Geometry check sheet. Reference: the model listing, model coordinates, mm. Face numbers are marked on the shaded views. A direction names the side the tool comes from. Coordinates: 2 decimals unless noted, no trailing zeros. Loops run counter-clockwise (first coordinate to the right, second up) from the corner with the lowest first, then second, coordinate; pieces in that order, holes last. Notation, with made-up numbers: M 12.5,-27 L 31.5,-27 A5 cw 31.5,-22 Z; hole C 66,-2 d8. An arc over 180 degrees is marked long. Use CSV: the item, a comma, the result in double quotes.
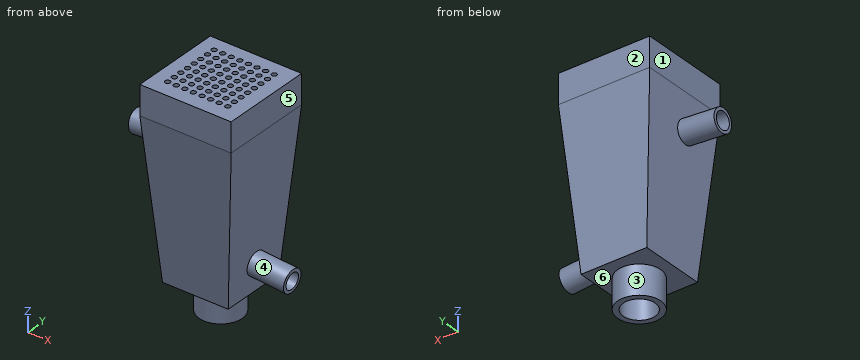
```python
from build123d import *

# Parameters (mm, degrees)
SKETCH2_4_W         = 25
SKETCH2_4_H         = 25
BOSS_EXTRUDE2_DEPTH = 8
SKETCH5_R           = 0.7
CUT_EXTRUDE1_DEPTH  = 8
SKETCH6_R           = 3.1
SKETCH6_R_2         = 2.3
BOSS_EXTRUDE4_DEPTH = 10
CUT_EXTRUDE2_START  = -4
SKETCH6_4_R         = 2.3
CUT_EXTRUDE2_DEPTH  = 4
SKETCH9_R           = 3.1
SKETCH9_R_2         = 2.2
BOSS_EXTRUDE5_DEPTH = 10
SKETCH1_7_R         = 5.88
SKETCH1_7_R_2       = 4.38
BOSS_EXTRUDE7_DEPTH = 8
CUT_EXTRUDE3_START  = -20
SKETCH10_R          = 2.2
CUT_EXTRUDE3_DEPTH  = 20


with BuildPart() as part:
    # Sketch1 → Loft1 section 0
    with BuildSketch(Plane.XY):
        with BuildLine():
            Line((-9, 9), (9, 9))
            Line((9, 9), (9, -9))
            Line((9, -9), (-9, -9))
            Line((-9, -9), (-9, 9))
        make_face()
    # Sketch2 → Loft1 section 1
    with BuildSketch(Plane.XY.offset(43)):
        with BuildLine():
            Line((-12.5, 12.5), (12.5, 12.5))
            Line((12.5, 12.5), (12.5, -12.5))
            Line((12.5, -12.5), (-12.5, -12.5))
            Line((-12.5, -12.5), (-12.5, 12.5))
        make_face()
    loft()

    # Cut-Loft1: read off the stored shape, not the designer's step
    # Cut-Loft1: loft between two sections, ruled curve by curve
    cut_loft1_from = [
        Edge.make_bspline([(-3.097127702, -3.097127702, 0), (-2.732127702, -3.462127702, 0), (-2.271815958, -3.789394651, 0), (-1.207457606, -4.2500242, 0), (-0.604751801, -4.38, 0), (0.604751801, -4.38, 0), (1.207457606, -4.2500242, 0), (2.271815958, -3.789394651, 0), (2.732127702, -3.462127702, 0), (3.097127702, -3.097127702, 0)], [0, 0, 0, 0, 0.25, 0.25, 0.5, 0.5, 0.75, 0.75, 1, 1, 1, 1], 3),
        Edge.make_bspline([(3.097127702, -3.097127702, 0), (3.462127702, -2.732127702, 0), (3.789394651, -2.271815958, 0), (4.2500242, -1.207457606, 0), (4.38, -0.604751801, 0), (4.38, 0.604751801, 0), (4.2500242, 1.207457606, 0), (3.789394651, 2.271815958, 0), (3.462127702, 2.732127702, 0), (3.097127702, 3.097127702, 0)], [0, 0, 0, 0, 0.25, 0.25, 0.5, 0.5, 0.75, 0.75, 1, 1, 1, 1], 3),
        Edge.make_bspline([(-3.097127702, 3.097127702, 0), (-3.462127702, 2.732127702, 0), (-3.789394651, 2.271815958, 0), (-4.2500242, 1.207457606, 0), (-4.38, 0.604751801, 0), (-4.38, -0.604751801, 0), (-4.2500242, -1.207457606, 0), (-3.789394651, -2.271815958, 0), (-3.462127702, -2.732127702, 0), (-3.097127702, -3.097127702, 0)], [0, 0, 0, 0, 0.25, 0.25, 0.5, 0.5, 0.75, 0.75, 1, 1, 1, 1], 3),
        Edge.make_bspline([(3.097127702, 3.097127702, 0), (2.732127702, 3.462127702, 0), (2.271815958, 3.789394651, 0), (1.207457606, 4.2500242, 0), (0.604751801, 4.38, 0), (-0.604751801, 4.38, 0), (-1.207457606, 4.2500242, 0), (-2.271815958, 3.789394651, 0), (-2.732127702, 3.462127702, 0), (-3.097127702, 3.097127702, 0)], [0, 0, 0, 0, 0.25, 0.25, 0.5, 0.5, 0.75, 0.75, 1, 1, 1, 1], 3),
    ]
    cut_loft1_to = [
        Edge.make_bspline([(-10, -10, 43), (-8.333333333, -10, 43), (-6.666666667, -10, 43), (-3.333333333, -10, 43), (-1.666666667, -10, 43), (1.666666667, -10, 43), (3.333333333, -10, 43), (6.666666667, -10, 43), (8.333333333, -10, 43), (10, -10, 43)], [0, 0, 0, 0, 0.25, 0.25, 0.5, 0.5, 0.75, 0.75, 1, 1, 1, 1], 3),
        Edge.make_bspline([(10, -10, 43), (10, -8.333333333, 43), (10, -6.666666667, 43), (10, -3.333333333, 43), (10, -1.666666667, 43), (10, 1.666666667, 43), (10, 3.333333333, 43), (10, 6.666666667, 43), (10, 8.333333333, 43), (10, 10, 43)], [0, 0, 0, 0, 0.25, 0.25, 0.5, 0.5, 0.75, 0.75, 1, 1, 1, 1], 3),
        Edge.make_bspline([(-10, 10, 43), (-10, 8.333333333, 43), (-10, 6.666666667, 43), (-10, 3.333333333, 43), (-10, 1.666666667, 43), (-10, -1.666666667, 43), (-10, -3.333333333, 43), (-10, -6.666666667, 43), (-10, -8.333333333, 43), (-10, -10, 43)], [0, 0, 0, 0, 0.25, 0.25, 0.5, 0.5, 0.75, 0.75, 1, 1, 1, 1], 3),
        Edge.make_bspline([(10, 10, 43), (8.333333333, 10, 43), (6.666666667, 10, 43), (3.333333333, 10, 43), (1.666666667, 10, 43), (-1.666666667, 10, 43), (-3.333333333, 10, 43), (-6.666666667, 10, 43), (-8.333333333, 10, 43), (-10, 10, 43)], [0, 0, 0, 0, 0.25, 0.25, 0.5, 0.5, 0.75, 0.75, 1, 1, 1, 1], 3),
    ]
    cut_loft1 = Solid(Shell([*[Face.make_surface_from_curves(cut_loft1_from[k], cut_loft1_to[k]) for k in range(4)], Face(Wire(cut_loft1_from)), Face(Wire(cut_loft1_to))]))
    add(cut_loft1, mode=Mode.SUBTRACT)

    # Sketch2<4> → Boss-Extrude2 (add)
    with BuildSketch(Plane.XY.offset(43)):
        Rectangle(SKETCH2_4_W, SKETCH2_4_H)
    extrude(amount=BOSS_EXTRUDE2_DEPTH)

    # Sketch5 → Cut-Extrude1 (cut)
    with BuildSketch(Plane.XY.offset(43)):
        with Locations((-8.388056057, 8.509622087)):
            Circle(SKETCH5_R)
        with Locations((-6.038056057, 8.509622087)):
            Circle(SKETCH5_R)
        with Locations((-3.688056057, 8.509622087)):
            Circle(SKETCH5_R)
        with Locations((-1.338056057, 8.509622087)):
            Circle(SKETCH5_R)
        with Locations((1.011943943, 8.509622087)):
            Circle(SKETCH5_R)
        with Locations((3.361943943, 8.509622087)):
            Circle(SKETCH5_R)
        with Locations((5.711943943, 8.509622087)):
            Circle(SKETCH5_R)
        with Locations((8.061943943, 8.509622087)):
            Circle(SKETCH5_R)
        with Locations((-6.038056057, 6.159622087)):
            Circle(SKETCH5_R)
        with Locations((-3.688056057, 6.159622087)):
            Circle(SKETCH5_R)
        with Locations((-1.338056057, 6.159622087)):
            Circle(SKETCH5_R)
        with Locations((1.011943943, 6.159622087)):
            Circle(SKETCH5_R)
        with Locations((3.361943943, 6.159622087)):
            Circle(SKETCH5_R)
        with Locations((5.711943943, 6.159622087)):
            Circle(SKETCH5_R)
        with Locations((8.061943943, 6.159622087)):
            Circle(SKETCH5_R)
        with Locations((-6.038056057, 3.809622087)):
            Circle(SKETCH5_R)
        with Locations((-3.688056057, 3.809622087)):
            Circle(SKETCH5_R)
        with Locations((-1.338056057, 3.809622087)):
            Circle(SKETCH5_R)
        with Locations((1.011943943, 3.809622087)):
            Circle(SKETCH5_R)
        with Locations((3.361943943, 3.809622087)):
            Circle(SKETCH5_R)
        with Locations((5.711943943, 3.809622087)):
            Circle(SKETCH5_R)
        with Locations((8.061943943, 3.809622087)):
            Circle(SKETCH5_R)
        with Locations((-6.038056057, 1.459622087)):
            Circle(SKETCH5_R)
        with Locations((-3.688056057, 1.459622087)):
            Circle(SKETCH5_R)
        with Locations((-1.338056057, 1.459622087)):
            Circle(SKETCH5_R)
        with Locations((1.011943943, 1.459622087)):
            Circle(SKETCH5_R)
        with Locations((3.361943943, 1.459622087)):
            Circle(SKETCH5_R)
        with Locations((5.711943943, 1.459622087)):
            Circle(SKETCH5_R)
        with Locations((8.061943943, 1.459622087)):
            Circle(SKETCH5_R)
        with Locations((-6.038056057, -0.890377913)):
            Circle(SKETCH5_R)
        with Locations((-3.688056057, -0.890377913)):
            Circle(SKETCH5_R)
        with Locations((-1.338056057, -0.890377913)):
            Circle(SKETCH5_R)
        with Locations((1.011943943, -0.890377913)):
            Circle(SKETCH5_R)
        with Locations((3.361943943, -0.890377913)):
            Circle(SKETCH5_R)
        with Locations((5.711943943, -0.890377913)):
            Circle(SKETCH5_R)
        with Locations((8.061943943, -0.890377913)):
            Circle(SKETCH5_R)
        with Locations((-6.038056057, -3.240377913)):
            Circle(SKETCH5_R)
        with Locations((-3.688056057, -3.240377913)):
            Circle(SKETCH5_R)
        with Locations((-1.338056057, -3.240377913)):
            Circle(SKETCH5_R)
        with Locations((1.011943943, -3.240377913)):
            Circle(SKETCH5_R)
        with Locations((3.361943943, -3.240377913)):
            Circle(SKETCH5_R)
        with Locations((5.711943943, -3.240377913)):
            Circle(SKETCH5_R)
        with Locations((8.061943943, -3.240377913)):
            Circle(SKETCH5_R)
        with Locations((-6.038056057, -5.590377913)):
            Circle(SKETCH5_R)
        with Locations((-3.688056057, -5.590377913)):
            Circle(SKETCH5_R)
        with Locations((-1.338056057, -5.590377913)):
            Circle(SKETCH5_R)
        with Locations((1.011943943, -5.590377913)):
            Circle(SKETCH5_R)
        with Locations((3.361943943, -5.590377913)):
            Circle(SKETCH5_R)
        with Locations((5.711943943, -5.590377913)):
            Circle(SKETCH5_R)
        with Locations((8.061943943, -5.590377913)):
            Circle(SKETCH5_R)
        with Locations((-6.038056057, -7.940377913)):
            Circle(SKETCH5_R)
        with Locations((-3.688056057, -7.940377913)):
            Circle(SKETCH5_R)
        with Locations((-1.338056057, -7.940377913)):
            Circle(SKETCH5_R)
        with Locations((1.011943943, -7.940377913)):
            Circle(SKETCH5_R)
        with Locations((3.361943943, -7.940377913)):
            Circle(SKETCH5_R)
        with Locations((5.711943943, -7.940377913)):
            Circle(SKETCH5_R)
        with Locations((8.061943943, -7.940377913)):
            Circle(SKETCH5_R)
        with Locations((-8.388056057, 6.159622087)):
            Circle(SKETCH5_R)
        with Locations((-8.388056057, 3.809622087)):
            Circle(SKETCH5_R)
        with Locations((-8.388056057, 1.459622087)):
            Circle(SKETCH5_R)
        with Locations((-8.388056057, -0.890377913)):
            Circle(SKETCH5_R)
        with Locations((-8.388056057, -3.240377913)):
            Circle(SKETCH5_R)
        with Locations((-8.388056057, -5.590377913)):
            Circle(SKETCH5_R)
        with Locations((-8.388056057, -7.940377913)):
            Circle(SKETCH5_R)
    extrude(amount=CUT_EXTRUDE1_DEPTH, mode=Mode.SUBTRACT)

    # Sketch6 → Boss-Extrude4 (add)
    with BuildSketch(Plane(origin=(-8.940765615, 0, -0.727736736), x_dir=(-0.08112705090276601, 0, 0.9967037682339824), z_dir=(-0.9967037682339824, 0, -0.08112705090276602))):
        with Locations(Location((34.477535136, -1.520969622, 0), (0, 0, 180))):
            Circle(SKETCH6_R)
        with Locations((34.477535136, -1.520969622)):
            Circle(SKETCH6_R_2, mode=Mode.SUBTRACT)
    extrude(amount=BOSS_EXTRUDE4_DEPTH)

    # Sketch6<4> → Cut-Extrude2 (cut)
    with BuildSketch(Plane(origin=(-8.940765615, 0, -0.727736736), x_dir=(-0.08112705090276601, 0, 0.9967037682339824), z_dir=(-0.9967037682339824, 0, -0.08112705090276602)).offset(CUT_EXTRUDE2_START)):
        with Locations((34.477535136, -1.520969622)):
            Circle(SKETCH6_4_R)
    extrude(amount=CUT_EXTRUDE2_DEPTH, mode=Mode.SUBTRACT)

    # Sketch9 → Boss-Extrude5 (add)
    with BuildSketch(Plane(origin=(8.940765615, 0, -0.727736736), x_dir=(-0.08112705090276603, 0, -0.9967037682339824), z_dir=(0.9967037682339824, 0, -0.08112705090276605))):
        with Locations((-8.341303969, 0)):
            Circle(SKETCH9_R)
        with Locations((-8.341303969, 0)):
            Circle(SKETCH9_R_2, mode=Mode.SUBTRACT)
    extrude(amount=BOSS_EXTRUDE5_DEPTH)

    # Sketch1<7> → Boss-Extrude7 (add)
    with BuildSketch(Plane.XY):
        Circle(SKETCH1_7_R)
        Circle(SKETCH1_7_R_2, mode=Mode.SUBTRACT)
    extrude(amount=-BOSS_EXTRUDE7_DEPTH)

    # Sketch10 → Cut-Extrude3 (cut)
    with BuildSketch(Plane(origin=(18.907803297, 0, -1.539007245), x_dir=(-0.08112705090276605, 0, -0.9967037682339824), z_dir=(0.9967037682339824, 0, -0.08112705090276606)).offset(CUT_EXTRUDE3_START)):
        with Locations((-8.341303969, 0)):
            Circle(SKETCH10_R)
    extrude(amount=CUT_EXTRUDE3_DEPTH, mode=Mode.SUBTRACT)


solid = part.part
```
1. Gauge pin test, flat ends, axial feed: P1, Ø0.8, axis at x = -3.69, y = -5.59, coming from the -Z side; P2, Ø4, axis at x = 0.5, z = 20.5, coming from the -Y side; P3, Ø1.6, axis at x = -6.04, y = 3.81, coming from the +Z side; P4, Ø6, axis at y = -7, z = 16, coming from the -X side. Record the tip position at first contact, or that the pin passes through.
The answers:
P1,"z = 0"
P2,"y = -10.83"
P3,"z = 51"
P4,"x = -10.55"
2. Section check A-A, the plane x = 8. Count the separate pieces of the cut face and the enclosed holes in it, plus the area to 3 significant figures.
The answers:
separate pieces,"8"
enclosed holes,"1"
area,"767 mm^2"
3. Set-up check for the marked faces 1, 2 and 3: record each of +Z, -Z, +X, -X, +Y, -Y from which the full face is reachable in a straight line by a thin tool's end or side.
The answers:
face 1,"+Z, -X, +Y, -Y"
face 2,"+Z, -Z, +X, -X, +Y"
face 3,"-Z"
4. Release check for a two-part mould opening along Z. For the marked faces 4, 5 and 6 record: +Z half, -Z half, draft (parallel to the pull), parting line (faces both ways), or undercut.
The answers:
face 4,"undercut"
face 5,"draft"
face 6,"-Z half"
5. Thickness scan on line 1 (Y direction, x = -12.5, z = 32.5); line 2 (Y direction, x = 5.5, z = 36.5); line 3 (Z direction, x = 2.5, y = -0.5). Record the ranges inside material, lowest first. Write a range as [from, to].
The answers:
line 1,"[-4.43, -3.56], [0.51, 1.39]"
line 2,"[-11.97, -9.07], [9.07, 11.97]"
line 3,"[43, 51]"
6. Section check B-B, the plane z = -2.5. Record the cut outline in (x, y), plus the area to 3 significant figures.
The answers:
outline,"C 0,0 d11.76; hole C 0,0 d8.76"
area,"48.3 mm^2"
